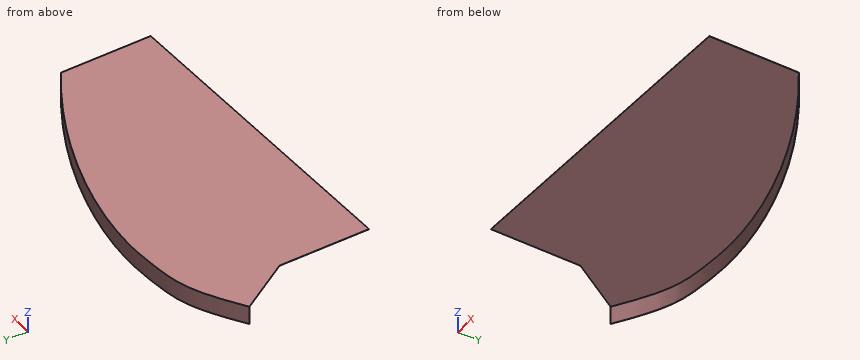
```python
from build123d import *

# Parameters (mm, degrees)
BOSS_EXTRUDE1_DEPTH = 0.1
BOSS_EXTRUDE2_DEPTH = 10


with BuildPart() as part:
    # Sketch1 → Boss-Extrude1 (new body)
    with BuildSketch(Plane.XY):
        with BuildLine():
            Line((-1544.649956659, 573.44143308), (-1542.397344254, 523.492201481))
            Line((-1542.397344254, 523.492201481), (-1721.722963635, 515.404967666))
            Line((-1721.722963635, 515.404967666), (-1723.97557604, 565.354199265))
            Line((-1723.97557604, 565.354199265), (-1743.607960183, 593.830470178))
            add(Edge.make_bspline(
                [(-1743.607960183, 593.830470178), (-1719.507904213, 610.537812828), (-1709.389541143, 613.399774739), (-1646.280289738, 619.241808081), (-1585.716648888, 600.423930323), (-1544.649956659, 573.44143308)],
                knots=[0, 0, 0, 0, 0.320554642, 0.420554642, 1, 1, 1, 1], degree=3))
        make_face()
    extrude(amount=BOSS_EXTRUDE1_DEPTH)

    # Sketch2 → Boss-Extrude2 (add)
    with BuildSketch(Plane.XY.offset(0.1)):
        with BuildLine():
            Line((-1544.677412579, 573.399645851), (-1544.732324417, 573.316071394))
            add(Edge.make_bspline(
                [(-1544.732324417, 573.316071394), (-1546.951948835, 574.774455463), (-1551.43127801, 577.613556033), (-1560.629429442, 583.045346231), (-1572.470935952, 589.326889692), (-1587.069867375, 596.019330748), (-1606.812651261, 603.755089396), (-1626.620904389, 609.625271881), (-1645.785452529, 613.461587482), (-1659.664022733, 615.275078476), (-1672.855430865, 616.000525973), (-1683.17584634, 615.607177853), (-1690.719151522, 614.940047919), (-1697.619410573, 614.184343593), (-1704.94143994, 613.175751133), (-1711.537062872, 611.520585877), (-1716.950731756, 609.496349748), (-1721.226339774, 607.54713974), (-1725.861820037, 605.087085053), (-1730.144377714, 602.544994912), (-1733.894814235, 600.175895508), (-1736.886084267, 598.222624564), (-1739.548362017, 596.435520579), (-1741.775682708, 594.914415574), (-1742.945821332, 594.106977842), (-1743.522500251, 593.707195687)],
                knots=[0, 0, 0, 0, 0.03125, 0.0625, 0.125, 0.1875, 0.25, 0.375, 0.4375, 0.5, 0.5625, 0.625, 0.65625, 0.6875, 0.75, 0.8125, 0.84375, 0.875, 0.90625, 0.9375, 0.953125, 0.96875, 0.984375, 0.9921875, 1, 1, 1, 1], degree=3))
            Line((-1743.522500251, 593.707195687), (-1743.579473539, 593.789378681))
            add(Edge.make_bspline(
                [(-1544.677412579, 573.399645851), (-1580.106306882, 596.677879158), (-1623.417276611, 611.817205851), (-1664.055554326, 615.615316249), (-1668.458587485, 615.853546332), (-1674.850456886, 615.924640206), (-1676.947072346, 615.898899542), (-1681.053950245, 615.760083504), (-1685.070934683, 615.538033819), (-1688.841535286, 615.206941309), (-1692.455660822, 614.85004283), (-1694.182553399, 614.660043123), (-1699.092177305, 614.084892783), (-1702.026740338, 613.678931579), (-1710.391454065, 612.076086015), (-1715.382812403, 610.494610736), (-1727.278520434, 604.6086441), (-1734.182625539, 600.30373531), (-1743.579473539, 593.789378681)],
                knots=[0, 0, 0, 0, 0.5, 0.5, 0.5625, 0.5625, 0.59375, 0.59375, 0.625, 0.65625, 0.65625, 0.6875, 0.6875, 0.75, 0.75, 0.875, 0.875, 1, 1, 1, 1], degree=3))
        make_face()
    extrude(amount=-BOSS_EXTRUDE2_DEPTH)


solid = part.part
```
Input: part model. Units: mm. Frame: model coordinates. Coordinates: 2 decimals unless noted, no trailing zeros. Write each loop counter-clockwise with the first axis right and the second up, starting at its lowest first coordinate (ties: lowest second). Pieces come first, ordered by that corner, then holes. Notation, with made-up numbers: (45, 83) - (63, 83) arc R15 ccw to (63, 111) - close; hole circle Ø6 at (69, 11.5). An arc over 180 degrees is marked (long way). Put each result on its own line as item: value. Start each with the question number.
1) Ray query, L1, parallel to X at y = 594, z = -7.5; L2, parallel to X at y = 595, z = -4.75; L3, parallel to X at y = 584, z = -3.75. Return the intervals inside material, ascending.
2) Contact query for flat-ended pins moving along their axis: pin 1 (3 mm diameter, centred on x = -1682.5, z = -8, fed in from -Y); pin 2 (3 mm diameter, centred on y = 578, z = -4, fed in from +X); pin 3 (12 mm diameter, centred on x = -1681.5, y = 589.5, fed in from -Z). Output: stop coordinate, or through.
3) Cut plane A-A (y = 542). Return the cut outline in (x, z), plus the area to 3 significant figures.
Resolved:
1. L1: x = -1743.28 to -1743.1, -1582.8 to -1582.55
1. L2: x = -1741.82 to -1741.65, -1585.08 to -1584.83
1. L3: x = -1562.56 to -1562.35
2. pin 1: stops at y = 615.48
2. pin 2: stops at x = -1549.52
2. pin 3: stops at z = 0
3. outline: (-1722.92, 0) - (-1543.23, 0) - (-1543.23, 0.1) - (-1722.92, 0.1) - close
3. area: 18.0 mm2
